Geometry check sheet. Reference: the model listing, model coordinates, mm. A direction names the side the tool comes from. Round coordinates to 2 decimals unless told otherwise and drop trailing zeros. Write each loop counter-clockwise with the first axis right and the second up, starting at its lowest first coordinate (ties: lowest second). Pieces come first, ordered by that corner, then holes. Notation, with made-up numbers: M 86,34.5 L 109,34.5 A32 cw 109,62.5 Z; hole C 39.5,32 d1. An arc over 180 degrees is marked long. One line per item, written item: value. Start each with the question number.
1. Scan lines: probe 1 along Z at (x, y) = (-20, -1); probe 2 along Z at (x, y) = (-5, 28.5); probe 3 along Y at (x, z) = (-2, 11.5). Record each from-to range of solid material in increasing order. Write a range as [from, to].
2. Section check A-A (z = 0). Record the boundary of the cut face in (x, y), and give its area (3 significant figures).
3. Section check B-B (z = 19). Record the boundary of the cut face in (x, y), and give its area (3 significant figures).
4. Depth check by flat-ended pin: P1, Ø5, axis at x = 8.5, z = -2, coming from the +Y side; P2, Ø2.5, axis at x = -10, y = 31.93, coming from the -Z side; P3, Ø10, axis at y = 7.5, z = 0.5, coming from the +X side. Enter the tip coordinate at first touch or a pass-through.
5. Access from +Z, -Z, +X, -X, +Y, -Y to the whole of each face (thin tool, end or side, straight path). Record for faces 1 (the flat face through (11, 0, 0)), 2 (the cylindrical face through (2.17, -0.99, -9.76)), 3 (the cylindrical face through (-9.8, 16.58, -24.99)), 4 (the cylindrical face through (-7.6, 29.5, 26)).
6. Section check D-D (y = 6). Record the boundary of the cut face in (x, z), and give its area (3 significant figures).
7. Release check for a two-part mould opening along X. For faces 5 (the cylindrical face through (-17.01, 23.513, -24.986)), 6 (the flat face through (25, -1, 1)), 7 (the flat face through (-5, 13, 28)), 8 (the flat face through (-22.933, 15.873, -24.986)) record: pulls with the +X half, pulls with the -X half, needs draft (parallel to the pull), parting line crosses it, or undercut.
8. Section check C-C (x = 4). Record the boundary of the cut face in (y, z).
from build123d import *

# Parameters (mm, degrees)
SKETCH_W     = 50
SKETCH_H     = 48
SKETCH_R     = 1.5
SKETCH_R_2   = 10
PAD_DEPTH    = 2
SKETCH003_R  = 1.5
PAD001_DEPTH = 2
SKETCH004_R  = 5.1
PAD002_DEPTH = 4
FILLET_R     = 1.99
FILLET001_R  = 1.99


with BuildPart() as body:
    # Sketch → Pad (new body)
    with BuildSketch(Plane.XZ):
        Rectangle(SKETCH_W, SKETCH_H)
        with Locations((-20, 19)):
            Circle(SKETCH_R, mode=Mode.SUBTRACT)
        with Locations((20, 19)):
            Circle(SKETCH_R, mode=Mode.SUBTRACT)
        with Locations((-20, -19)):
            Circle(SKETCH_R, mode=Mode.SUBTRACT)
        with Locations((20, -19)):
            Circle(SKETCH_R, mode=Mode.SUBTRACT)
        Circle(SKETCH_R_2, mode=Mode.SUBTRACT)
    extrude(amount=PAD_DEPTH)

    # Sketch003 (on Face3 of Pad) → Pad001 (join)
    with BuildSketch(Plane(origin=(0, 0, -24), x_dir=(1, 0, 0), z_dir=(0, 0, -1))):
        with BuildLine():
            Line((-25, 0), (-25, 2))
            Line((-25, 2), (25, 2))
            Line((25, 2), (25, 0))
            Line((25, 0), (25, -5))
            Line((25, -5), (20.80638, -27.054785))
            ThreePointArc((1.756653, -32.283353), (12.911489, -35.607697), (20.80638, -27.054785))
            Line((-25, -2), (1.756653, -32.283353))
            Line((-25, 0), (-25, -2))
        make_face()
        with Locations((10, -31.934549)):
            Circle(SKETCH003_R, mode=Mode.SUBTRACT)
        with Locations((17.205, -25)):
            Circle(SKETCH003_R, mode=Mode.SUBTRACT)
        with Locations((10, -25)):
            Circle(SKETCH003_R, mode=Mode.SUBTRACT)
        with Locations((2.795, -25)):
            Circle(SKETCH003_R, mode=Mode.SUBTRACT)
        with Locations((10, -18.065451)):
            Circle(SKETCH003_R, mode=Mode.SUBTRACT)
    extrude(amount=PAD001_DEPTH)

    # Sketch004 (on Face1 of Pad) → Pad002 (join)
    with BuildSketch(Plane(origin=(0, 0, 24), x_dir=(-1, 0, 0), z_dir=(0, 0, 1))):
        with BuildLine():
            Line((-25, 2), (25, 2))
            Line((25, 2), (25, 0))
            Line((25, 0), (25, -2))
            Line((25, -2), (-1.756653, -32.283353))
            ThreePointArc((-20.80638, -27.054785), (-12.911489, -35.607697), (-1.756653, -32.283353))
            Line((-25, -5), (-20.80638, -27.054785))
            Line((-25, 0), (-25, -5))
            Line((-25, 0), (-25, 2))
        make_face()
        with Locations((-10, -25)):
            Circle(SKETCH004_R, mode=Mode.SUBTRACT)
    extrude(amount=PAD002_DEPTH)

    # Fillet
    fillet_edges = [body.edges().sort_by_distance(p)[0] for p in [
        (0, 0, 24),
    ]]
    fillet(fillet_edges, radius=FILLET_R)

    # Fillet001
    fillet001_edges = [body.edges().sort_by_distance(p)[0] for p in [
        (0, 0, -24),
    ]]
    fillet(fillet001_edges, radius=FILLET001_R)


with BuildPart() as part_mirroring:
    # Part__Mirroring: instance of Body
    add(body.part.mirror(Plane(origin=(0, 0, 0), x_dir=(0, -1, 0), z_dir=(1, 0, 0))))


solid = part_mirroring.part
Result sheet:
1. probe 1: z = [-26, -20.5], [-17.5, 17.5], [20.5, 28]
1. probe 2: z = [-26, -24], [24, 28]
1. probe 3: y = [-2, 0]
2. outline: M -25,-2 L -10,-2 L -10,0 L -25,0 Z; M 10,-2 L 25,-2 L 25,0 L 10,0 Z
2. area: 60.0 mm2
3. outline: M -25,-2 L -21.5,-2 L -21.5,0 L -25,0 Z; M -18.5,-2 L 18.5,-2 L 18.5,0 L -18.5,0 Z; M 21.5,-2 L 25,-2 L 25,0 L 21.5,0 Z
3. area: 88.0 mm2
4. P1: stops at y = 0
4. P2: stops at z = 24
4. P3: passes through
5. face 1: +X, -X, +Y
5. face 2: +Y, -Y
5. face 3: -Z
5. face 4: +Z
6. outline: M -24.81,-26 L 21.47,-26 L 21.47,-24 L -24.81,-24 Z; M -24.81,24 L 21.47,24 L 21.47,28 L -24.81,28 Z
6. area: 278 mm2
7. face 5: undercut
7. face 6: pulls with the +X half
7. face 7: needs draft
7. face 8: pulls with the -X half
8. outline: M -2,-26 L 25.77,-26 L 25.77,-24 L 1.99,-24 A1.99 cw 0,-22.01 L 0,-9.17 L -2,-9.17 Z; M -2,9.17 L 0,9.17 L 0,22.01 A1.99 cw 1.99,24 L 25.77,24 L 25.77,28 L -2,28 Z
